Build history of the part. All positions in model axes, mm. Face numbers are marked on the shaded views. Round coordinates to 2 decimals unless told otherwise and drop trailing zeros. Write each loop counter-clockwise with the first axis right and the second up, starting at its lowest first coordinate (ties: lowest second). Pieces come first, ordered by that corner, then holes.
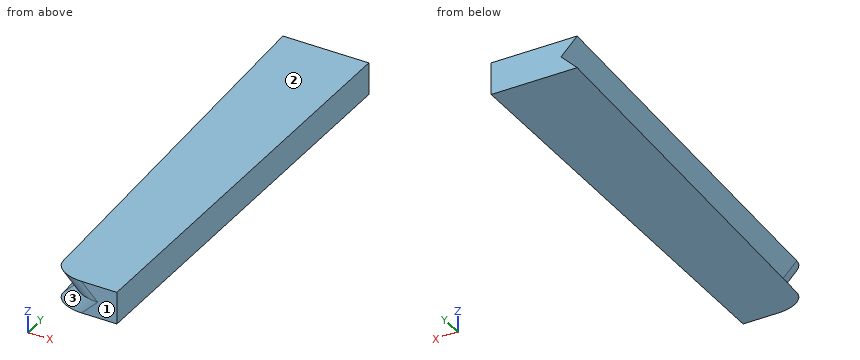
from build123d import *

# Parameters (mm, degrees)
F1_DEPTH     = 200
F2_T1_DEPTH  = 531.7746698901
F2_T3_DEPTH  = 531.7746698901
F2_T9_DEPTH  = 1052.9427380625
F2_T14_DEPTH = 1052.9427380625
F3_R         = 10


# Not quite as in the source:
# - a fillet or chamfer that OpenCascade refuses, or shapes differently, is made with other operations: its cross-section is extruded or revolved along the edge and cut away or added


with BuildPart() as f1:
    # F0 (on Front) → F1 (new body)
    with BuildSketch(Plane.XZ):
        Polygon((-25, 0), (0, 0), (0, 15), (-40, 15), (-32.5, 7.5), (-40, 0), align=None)
    extrude(amount=F1_DEPTH)

    # F2: chamfer of 7 x 200.4537729804 on 2 edges, made by hand

    # F2_s2 → F2_t1 (cut)
    with BuildSketch(Plane(origin=(-396.0214751426, 0, 396.0214751426), x_dir=(0, 1, 0), z_dir=(0.7071067812, 0, -0.7071067812))):
        Polygon((-200, -10.6776695297), (0.4537729804, -17.6776695297), (-200, -17.6776695297), align=None)
    extrude(amount=F2_T1_DEPTH, mode=Mode.SUBTRACT)

    # F2_s4 → F2_t3 (cut)
    with BuildSketch(Plane(origin=(-12.5, 0, -12.5), x_dir=(0, 1, 0), z_dir=(-0.7071067812, 0, -0.7071067812))):
        Polygon((-200, -21.2842712475), (0.4537729804, -28.2842712475), (-200, -28.2842712475), align=None)
    extrude(amount=F2_T3_DEPTH, mode=Mode.SUBTRACT)


with BuildPart() as f2_tool7:
    # F2_s8 → F2_t9 (new body)
    with BuildSketch(Plane(origin=(-396.0214751426, 0, 396.0214751426), x_dir=(0, 1, 0), z_dir=(0.7071067812, 0, -0.7071067812))):
        Polygon((-200, -10.6776695297), (0.4537729804, -17.6776695297), (-200, -17.6776695297), align=None)
    extrude(amount=F2_T9_DEPTH)

    split(bisect_by=Plane.XY, keep=Keep.TOP)

    split(bisect_by=Plane(origin=(-20, 0, 20), x_dir=(0, 1, 0), z_dir=(0.7071067812, 0, -0.7071067812)), keep=Keep.TOP)


with BuildPart() as f2_tool12:
    # F2_s13 → F2_t14 (new body)
    with BuildSketch(Plane(origin=(356.0214751426, 0, 356.0214751426), x_dir=(0, 1, 0), z_dir=(-0.7071067812, 0, -0.7071067812))):
        Polygon((-200, -21.2842712475), (0.4537729804, -28.2842712475), (-200, -28.2842712475), align=None)
    extrude(amount=F2_T14_DEPTH)

    split(bisect_by=Plane(origin=(-12.5, 0, -12.5), x_dir=(0, 1, 0), z_dir=(0.7071067812, 0, 0.7071067812)), keep=Keep.TOP)

    split(bisect_by=Plane.XY.offset(15), keep=Keep.BOTTOM)


with BuildPart() as f2_tool7_1:
    add(f2_tool7.part)

    # F2_t17: intersect F2_tool12
    add(f2_tool12.part, mode=Mode.INTERSECT)


with BuildPart() as f1_1:
    add(f1.part)

    # F2_t5: cut F2_tool7
    add(f2_tool7_1.part, mode=Mode.SUBTRACT)

    # F3
    f3_edges = [f1_1.edges().sort_by_distance(p)[0] for p in [
        (-26.350505, -200, 11.25),
        (-26.350505, -200, 3.75),
    ]]
    fillet(f3_edges, radius=F3_R)


solid = f1_1.part
1) Mould opens along Z. For the marked faces 1, 2 and 3 say: released by +Z, released by -Z, zero draft, split by the parting line, or undercut.
Results:
face 1: zero draft
face 2: released by +Z
face 3: undercut
2) Wall check: L1, parallel to X at y = -187.5, z = 5; L2, parallel to Z at x = -25, y = -191; L3, parallel to Y at x = -18, z = 1.5. Give the ranges that are in metal, low to high.
Results:
L1: x = -25.72 to 0
L2: z = 0 to 5.51, 9.49 to 15
L3: y = -199.76 to 0
3) Slice it at B-B (y = -166). Write the cut outline in (x, z).
Results:
outline: (-31.78, 0) - (0, 0) - (0, 15) - (-31.78, 15) - (-24.28, 7.5) - close
4) Slice it at A-A (x = -36). Write the cut outline in (y, z), plus the area to 3 significant figures.
Results:
outline: (-80.54, 0) - (0, 0) - (0, 3.98) - close; (-80.54, 15) - (0, 11.02) - (0, 15) - close
area: 320 mm2
5) Slice it at C-C (y = -61). Write the cut outline in (x, z), plus the area to 3 significant figures.
Results:
outline: (-36.97, 0) - (0, 0) - (0, 15) - (-36.97, 15) - (-29.47, 7.5) - close
area: 498 mm2
